The listing builds one solid part. Answer for the finished solid, in the listing's coordinates (mm). A direction names the side the tool comes from. Coordinates: 2 decimals unless noted, no trailing zeros. Loops run counter-clockwise (first coordinate to the right, second up) from the corner with the lowest first, then second, coordinate; pieces in that order, holes last. Notation, with made-up numbers: (89.5, 75.25) - (107.5, 75.25) arc R35 ccw to (107.5, 107.25) - close; hole circle Ø1 at (88.25, -10.75). An arc over 180 degrees is marked (long way). One line per question, with ' | ' between items.
from build123d import *

# Parameters (mm, degrees)
SKETCH1_R           = 4.5
BOSS_EXTRUDE1_DEPTH = 5
SKETCH2_W           = 20
SKETCH2_H           = 29.3
BOSS_EXTRUDE2_DEPTH = 25
CUT_EXTRUDE1_DEPTH  = 30
SKETCH4_R           = 2.5
SKETCH4_R_2         = 3
CUT_EXTRUDE2_DEPTH  = 30
FILLET2_R           = 1


with BuildPart() as part:
    # Sketch1 → Boss-Extrude1 (new body)
    with BuildSketch(Plane.XY):
        Polygon((-10, 10), (-10, -10), (10, -10), (10, 10), (10, 39.3), (-10, 39.3), align=None)
        Circle(SKETCH1_R, mode=Mode.SUBTRACT)
    extrude(amount=BOSS_EXTRUDE1_DEPTH)

    # Sketch2 → Boss-Extrude2 (add)
    with BuildSketch(Plane(origin=(0, 0, 0), x_dir=(-1, 0, 0), z_dir=(0, 0, -1))):
        with Locations((0, 24.65)):
            Rectangle(SKETCH2_W, SKETCH2_H)
    extrude(amount=BOSS_EXTRUDE2_DEPTH)

    # Sketch3 → Cut-Extrude1 (cut)
    with BuildSketch(Plane(origin=(10, 0, 0), x_dir=(0, 0, -1), z_dir=(1, 0, 0))):
        Polygon((0, 15), (-5, 15), (-5, 39.3), (20, 39.3), (20, 15), align=None)
    extrude(amount=-CUT_EXTRUDE1_DEPTH, mode=Mode.SUBTRACT)

    # Sketch4 → Cut-Extrude2 (cut)
    with BuildSketch(Plane.XY.offset(-20)):
        with Locations((0, 45)):
            Circle(SKETCH4_R)
        with Locations((0, 25)):
            Circle(SKETCH4_R_2)
    extrude(amount=-CUT_EXTRUDE2_DEPTH, mode=Mode.SUBTRACT)

    # Fillet2
    fillet2_edges = [part.edges().sort_by_distance(p)[0] for p in [
        (-10, 39.3, -22.5),
        (10, 39.3, -22.5),
        (0, 15, -20),
        (0, 15, 5),
    ]]
    fillet(fillet2_edges, radius=FILLET2_R)


solid = part.part
Item 1: The mould has two halves that part along X. Classify faces 4 (the face through (-9.699, 39.015, -22.465)), 5 (the face through (-0.65, 22.07, -22.46)), 6 (the face through (0, 15, -7)): pulls with the +X half, pulls with the -X half, needs draft (parallel to the pull), parting line crosses it, or undercut.
Taken from the geometry:
face 4: pulls with the -X half | face 5: undercut | face 6: needs draft
Item 2: Find the intervals of material crossed by line 1 (Y direction, x = 0, z = 3.6); line 2 (Y direction, x = 0, z = -23.3); line 3 (Y direction, x = 9, z = -10.5), in increasing order. Write a range as [from, to].
Taken from the geometry:
line 1: y = [-10, -4.5], [4.5, 15] | line 2: y = [10, 22], [28, 39.3] | line 3: y = [10, 15]
Item 3: Each of these flat-tipped pins is pushed along its axis until it touches: pin 1 Ø4 at (x, z) = (4.5, -16.5) entering from +Y; pin 2 Ø6 at (x, y) = (-4, 0.5) entering from -Z; pin 3 Ø1.5 at (x, z) = (4.5, -13) entering from -Y. Where does it stop, or does it pass through?
Taken from the geometry:
pin 1: stops at y = 15 | pin 2: stops at z = 0 | pin 3: stops at y = 10
Item 4: Find section D-D, the plane x = 6.25. Write down the section's boundary in (y, z), plus the area to 4 significant figures.
Taken from the geometry:
outline: (-10, 0) - (10, 0) - (10, -25) - (39.3, -25) - (39.3, -20) - (16, -20) arc R1 cw to (15, -19) - (15, 4) arc R1 ccw to (14, 5) - (-10, 5) - close | area: 371.5 mm2
Item 5: Find section A-A, the plane y = 0. Write down the section's boundary in (x, z).
Taken from the geometry:
outline: (-10, 0) - (-4.5, 0) - (-4.5, 5) - (-10, 5) - close; (4.5, 0) - (10, 0) - (10, 5) - (4.5, 5) - close
Item 6: Find section C-C, the plane z = 2.25. Write down the section's boundary in (x, y).
Taken from the geometry:
outline: (-10, -10) - (10, -10) - (10, 15) - (-10, 15) - close; hole circle Ø9 at (0, 0)
Item 7: Which of the six approach directions +Z, -Z, +X, -X, +Y, -Y give full straight-line access (tool end or side, diameter ignored) to faces 1 (the face through (0, 5, 0)), 2 (the face through (0, -10, 2)), 3 (the face through (2, 28, -20))?
Taken from the geometry:
face 1: -Z, +X, -X, -Y | face 2: +Z, -Z, +X, -X, -Y | face 3: +Z, +X, -X, +Y
Item 8: Find section B-B, the plane x = 0. Write down the section's boundary in (y, z), plus the area to 4 significant figures.
Taken from the geometry:
outline: (-10, 0) - (-4.5, 0) - (-4.5, 5) - (-10, 5) - close; (4.5, 0) - (10, 0) - (10, -25) - (22, -25) - (22, -20) - (16, -20) arc R1 cw to (15, -19) - (15, 4) arc R1 ccw to (14, 5) - (4.5, 5) - close; (28, -25) - (39.3, -25) - (39.3, -20) - (28, -20) - close | area: 296.5 mm2
